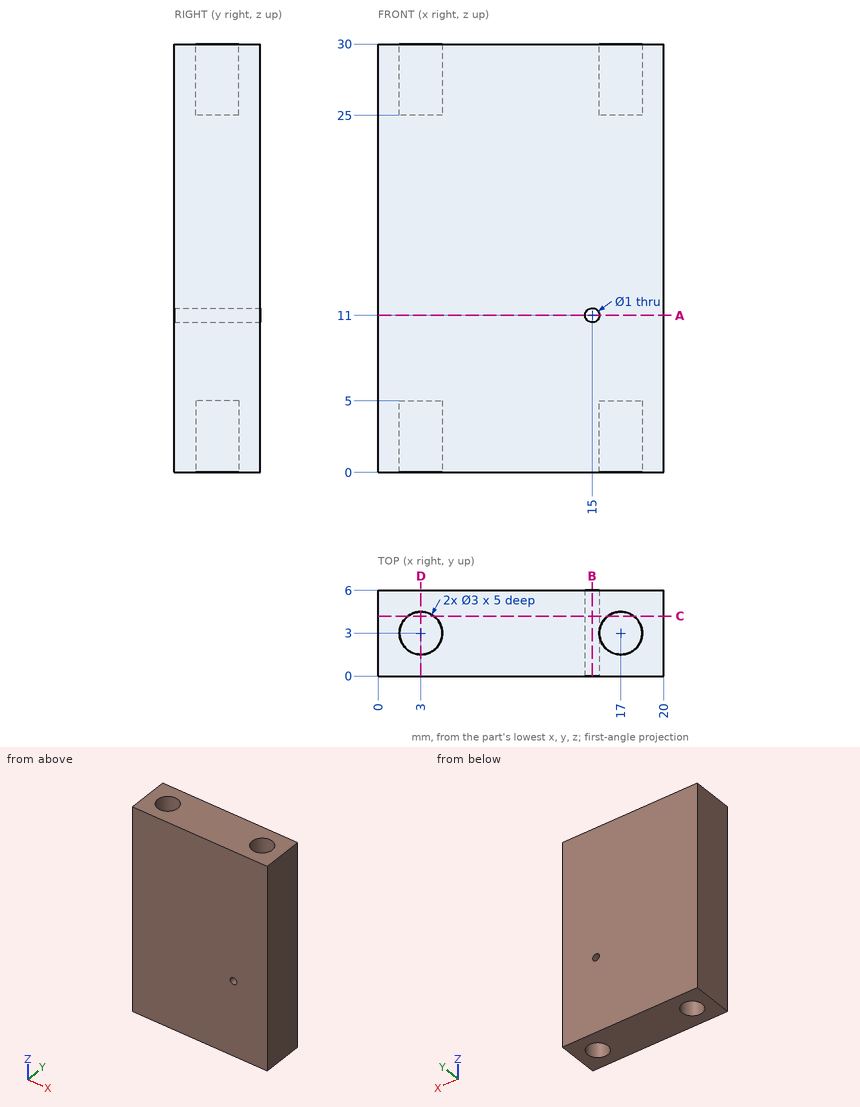
Input: dimensioned drawing with shaded views. Units: mm. Origin: part minimum x, y, z. Coordinates: 2 decimals unless noted, no trailing zeros. Write each loop counter-clockwise with the first axis right and the second up, starting at its lowest first coordinate (ties: lowest second). Pieces come first, ordered by that corner, then holes. Notation, with made-up numbers: M 36,5.5 L 61,5.5 A20 cw 61,43.5 Z; hole C 22.25,-2 d8. An arc over 180 degrees is marked long. Answer as CSV lines item,"result". Start each with the question number.
Q1. Pin query (flat end, axial travel): P1, Ø1.5, axis at x = 16.5, y = 2.5, coming from the -Z side; P2, Ø2.5, axis at x = 2.5, y = 3.5, coming from the +Z side; P3, Ø1.5, axis at x = 16.5, y = 3, coming from the +Z side. Return the tip coordinate at first contact, or that it passes through.
Q2. Line query: line 1 (Z direction, x = 15, y = 2.15); line 2 (Y direction, x = 17, z = 1.15). Output: solid intervals per line, ascending. Write a range as from..to.
Q3. Cut plane D-D on x = 3. Return the cut outline in (y, z).
Q4. Cut plane B-B on x = 15. Return the cut outline in (y, z), then the cut area to 3 significant figures.
Q5. Cut plane A-A on z = 11. Return the cut outline in (x, y).
Q6. Cut plane C-C on y = 4.2. Return the cut outline in (x, z).
Findings below:
1,P1,"stops at z = 5"
1,P2,"stops at z = 30"
1,P3,"stops at z = 25"
2,line 1,"z = 0..10.5, 11.5..30"
2,line 2,"y = 0..1.5, 4.5..6"
3,outline,"M 0,0 L 1.5,0 L 1.5,5 L 4.5,5 L 4.5,0 L 6,0 L 6,30 L 4.5,30 L 4.5,25 L 1.5,25 L 1.5,30 L 0,30 Z"
4,outline,"M 0,0 L 6,0 L 6,10.5 L 0,10.5 Z; M 0,11.5 L 6,11.5 L 6,30 L 0,30 Z"
4,area,"174 mm2"
5,outline,"M 0,0 L 14.5,0 L 14.5,6 L 0,6 Z; M 15.5,0 L 20,0 L 20,6 L 15.5,6 Z"
6,outline,"M 0,0 L 2.1,0 L 2.1,5 L 3.9,5 L 3.9,0 L 16.1,0 L 16.1,5 L 17.9,5 L 17.9,0 L 20,0 L 20,30 L 17.9,30 L 17.9,25 L 16.1,25 L 16.1,30 L 3.9,30 L 3.9,25 L 2.1,25 L 2.1,30 L 0,30 Z; hole C 15,11 d1"
